from build123d import *

# Parameters (mm, degrees)
EXTRUDE_1_DEPTH = 5
SKETCH_2_W      = 15
SKETCH_2_H      = 15
SKETCH_2_R      = 0.5
EXTRUDE_2_DEPTH = 3


with BuildPart() as part:
    # Эскиз1 → Бобышка-Вытянуть1 (new body)
    with BuildSketch(Plane(origin=(0, 0, 0), x_dir=(0, 0, -1), z_dir=(1, 0, 0))):
        Polygon((-10, 20), (0, 0), (0, 20), align=None)
    extrude(amount=EXTRUDE_1_DEPTH)

    # Эскиз2 → Бобышка-Вытянуть2 (add)
    with BuildSketch(Plane(origin=(0, 20, 0), x_dir=(1, 0, 0), z_dir=(0, 1, 0))):
        with Locations((2.5, -5)):
            Rectangle(SKETCH_2_W, SKETCH_2_H)
        with Locations(Location((-2.5, -5, 0), (0, 0, 270))):
            Circle(SKETCH_2_R, mode=Mode.SUBTRACT)
        with Locations(Location((7.5, -5, 0), (0, 0, 270))):
            Circle(SKETCH_2_R, mode=Mode.SUBTRACT)
    extrude(amount=EXTRUDE_2_DEPTH)


solid = part.part
Build history of the part. All positions in model axes, mm. A direction names the side the tool comes from. Round coordinates to 2 decimals unless told otherwise and drop trailing zeros. Write each loop counter-clockwise with the first axis right and the second up, starting at its lowest first coordinate (ties: lowest second). Pieces come first, ordered by that corner, then holes. Notation, with made-up numbers: (60, 84.5) - (88, 84.5) arc R31 cw to (88, 119.5) - close; hole circle Ø3 at (65, -18). An arc over 180 degrees is marked (long way). Use CSV: the item, a comma, the result in double quotes.
(1) Band-saw the part on D-D (z = 9). Write the cut outline in (x, y).
Response:
outline,"(-5, 20) - (0, 20) - (0, 18) - (5, 18) - (5, 20) - (10, 20) - (10, 23) - (-5, 23) - close"
(2) Band-saw the part on A-A (x = 7.5). Write the cut outline in (y, z), plus the area to 3 significant figures.
Response:
outline,"(20, -2.5) - (23, -2.5) - (23, 4.5) - (20, 4.5) - close; (20, 5.5) - (23, 5.5) - (23, 12.5) - (20, 12.5) - close"
area,"42.0 mm²"
(3) Wall check: line 1 (X direction, y = 21.2, z = 5); line 2 (Y direction, x = 7, z = 2); line 3 (X direction, y = 14.75, z = 1). Give the ranges that are in metal, low to high.
Response:
line 1,"-5 to -3, -2 to 7, 8 to 10"
line 2,"20 to 23"
line 3,"0 to 5"
(4) Pin check, flat tips, straight feed: P1, Ø8, axis at x = 4.5, y = 6.5, coming from the +Z side; P2, Ø7.5, axis at x = 3, z = 7.5, coming from the -Y side; P3, Ø2.5, axis at x = 2.5, y = 14, coming from the -Z side. Stop position of each tip, or through.
Response:
P1,"z = 5.25"
P2,"y = 7.5"
P3,"z = 0"
(5) Band-saw the part on B-B (z = 5). Write the cut outline in (x, y).
Response:
outline,"(-5, 20) - (-3, 20) - (-3, 23) - (-5, 23) - close; (-2, 20) - (0, 20) - (0, 10) - (5, 10) - (5, 20) - (7, 20) - (7, 23) - (-2, 23) - close; (8, 20) - (10, 20) - (10, 23) - (8, 23) - close"
(6) 3-axis set-ups, long thin cutter, end or side, ignore diameter. For faces 1 (the flat face through (2, 10, 5)), 2 (the flat face through (2, 10, 0)), 3 (the flat face through (0, 15, 3)): which of +Z, -Z, +X, -X, +Y, -Y reach the whole face in a straight line?
Response:
face 1,"+Z, +X, -X, -Y"
face 2,"-Z, +X, -X, -Y"
face 3,"+Z, -Z, -X, -Y"
(7) Band-saw the part on C-C (x = 1.75). Write the cut outline in (y, z), plus the area to 3 significant figures.
Response:
outline,"(0, 0) - (20, 0) - (20, -2.5) - (23, -2.5) - (23, 12.5) - (20, 12.5) - (20, 10) - close"
area,"145 mm²"
(8) Mould opens along X. For faces 4 (the flat face through (5, 15, 3)), 5 (the flat face through (2, 21, -2.5)), 6 (the cylindrical face through (7, 21, 5)) say: pulls with the +X half, pulls with the -X half, needs draft (parallel to the pull), parting line crosses it, or undercut.
Response:
face 4,"pulls with the +X half"
face 5,"needs draft"
face 6,"undercut"
